Work out the finished part from the listing and answer in its coordinate system (mm). Coordinates: 2 decimals unless noted, no trailing zeros. Loops run counter-clockwise (first coordinate to the right, second up) from the corner with the lowest first, then second, coordinate; pieces in that order, holes last.
```python
from build123d import *

# Parameters (mm, degrees)
MODEL_R                 = 1.5
SALIENTE_EXTRUIR1_DEPTH = 3


with BuildPart() as part:
    # Model → Saliente-Extruir1 (new body)
    with BuildSketch(Plane.XY):
        Polygon((-105.943383637, 105.556539338), (-105.943383637, 42.556539338), (-42.943383637, 42.556539338), align=None)
        with Locations((-101.443383637, 92.056539338)):
            Circle(MODEL_R, mode=Mode.SUBTRACT)
        with Locations((-101.443383637, 83.056539338)):
            Circle(MODEL_R, mode=Mode.SUBTRACT)
        with Locations((-92.443383637, 83.056539338)):
            Circle(MODEL_R, mode=Mode.SUBTRACT)
        with Locations((-101.443383637, 74.056539338)):
            Circle(MODEL_R, mode=Mode.SUBTRACT)
        with Locations((-92.443383637, 74.056539338)):
            Circle(MODEL_R, mode=Mode.SUBTRACT)
        with Locations((-83.443383637, 74.056539338)):
            Circle(MODEL_R, mode=Mode.SUBTRACT)
        with Locations((-101.443383637, 65.056539338)):
            Circle(MODEL_R, mode=Mode.SUBTRACT)
        with Locations((-92.443383637, 65.056539338)):
            Circle(MODEL_R, mode=Mode.SUBTRACT)
        with Locations((-83.443383637, 65.056539338)):
            Circle(MODEL_R, mode=Mode.SUBTRACT)
        with Locations((-74.443383637, 65.056539338)):
            Circle(MODEL_R, mode=Mode.SUBTRACT)
        with Locations((-101.443383637, 56.056539338)):
            Circle(MODEL_R, mode=Mode.SUBTRACT)
        with Locations((-92.443383637, 56.056539338)):
            Circle(MODEL_R, mode=Mode.SUBTRACT)
        with Locations((-83.443383637, 56.056539338)):
            Circle(MODEL_R, mode=Mode.SUBTRACT)
        with Locations((-74.443383637, 56.056539338)):
            Circle(MODEL_R, mode=Mode.SUBTRACT)
        with Locations((-65.443383637, 56.056539338)):
            Circle(MODEL_R, mode=Mode.SUBTRACT)
        with Locations((-101.443383637, 47.056539338)):
            Circle(MODEL_R, mode=Mode.SUBTRACT)
        with Locations((-92.443383637, 47.056539338)):
            Circle(MODEL_R, mode=Mode.SUBTRACT)
        with Locations((-83.443383637, 47.056539338)):
            Circle(MODEL_R, mode=Mode.SUBTRACT)
        with Locations((-74.443383637, 47.056539338)):
            Circle(MODEL_R, mode=Mode.SUBTRACT)
        with Locations((-65.443383637, 47.056539338)):
            Circle(MODEL_R, mode=Mode.SUBTRACT)
        with Locations((-56.443383637, 47.056539338)):
            Circle(MODEL_R, mode=Mode.SUBTRACT)
    extrude(amount=SALIENTE_EXTRUIR1_DEPTH)


solid = part.part
```
1. A cutting plane is placed at B-B, the plane x = -92. Give the vertices of the cut face in (y, z), then the cut area to 3 significant figures.
2. A cutting plane is placed at A-A, the plane x = -66. Give the vertices of the cut face in (y, z), then the cut area to 3 significant figures.
3. A cutting plane is placed at D-D, the plane x = -56. Give the vertices of the cut face in (y, z).
4. Each of these flat-tipped pins is pushed along its axis until it touches: P1, Ø5, axis at x = -92.44, y = 47.06, coming from the -Z side; P2, Ø1.5, axis at x = -52, z = 1, coming from the +Y side; P3, Ø1, axis at y = 58.5, z = 0.5, coming from the +X side. Where does it stop, or does it pass through?
5. A cutting plane is placed at C-C, the plane z = 2.3. Count the separate pieces of the cut face and the enclosed holes in it, then the cut area to 3 significant figures.
6. Straight lines are drawn through the part: probe 1 along Y at (x, z) = (-66, 1); probe 2 along Y at (x, z) = (-66.5, 1.15); probe 3 along Y at (x, z) = (-74.5, 2.35). For each, find the intervals that lie inside material, in ascending order.
7. Determine the mould class of faces 1 (the cylindrical face through (-55.013, 47.507, 1.479)), 2 (the flat face through (-89, 60, 3)) for opening direction Y: released by +Y, released by -Y, zero draft, split by the parting line, or undercut.
Answers below:
1. outline: (42.56, 0) - (45.62, 0) - (45.62, 3) - (42.56, 3) - close; (48.49, 0) - (54.62, 0) - (54.62, 3) - (48.49, 3) - close; (57.49, 0) - (63.62, 0) - (63.62, 3) - (57.49, 3) - close; (66.49, 0) - (72.62, 0) - (72.62, 3) - (66.49, 3) - close; (75.49, 0) - (81.62, 0) - (81.62, 3) - (75.49, 3) - close; (84.49, 0) - (91.61, 0) - (91.61, 3) - (84.49, 3) - close
1. area: 104 mm2
2. outline: (42.56, 0) - (45.66, 0) - (45.66, 3) - (42.56, 3) - close; (48.45, 0) - (54.66, 0) - (54.66, 3) - (48.45, 3) - close; (57.45, 0) - (65.61, 0) - (65.61, 3) - (57.45, 3) - close
2. area: 52.5 mm2
3. outline: (42.56, 0) - (45.62, 0) - (45.62, 3) - (42.56, 3) - close; (48.49, 0) - (55.61, 0) - (55.61, 3) - (48.49, 3) - close
4. P1: stops at z = 0
4. P2: stops at y = 52.36
4. P3: stops at x = -58.39
5. separate pieces: 1
5. enclosed holes: 21
5. area: 1,840 mm2
6. probe 1: y = 42.56 to 45.66, 48.45 to 54.66, 57.45 to 65.61
6. probe 2: y = 42.56 to 45.99, 48.12 to 54.99, 57.12 to 66.11
6. probe 3: y = 42.56 to 45.56, 48.56 to 54.56, 57.56 to 63.56, 66.56 to 74.11
7. face 1: undercut
7. face 2: zero draft
